Autodesk Inventor part; units mm, degrees
ref_plane "YZ Plane" through (0, 0, 0) normal (1, 0, 0) x (0, 1, 0)
ref_plane "XZ Plane" through (0, 0, 0) normal (0, 1, 0) x (-1, 0, 0)
ref_plane "XY Plane" through (0, 0, 0) normal (0, 0, 1) x (1, 0, 0)
ref_plane "Work Plane1" through (0, 0, 0) normal (0, 0, 1) x (1, 0, 0)
sketch "Sketch1" plane through (0, 0, 0) normal (0, 0, 1) x (1, 0, 0)
  circle A0 centre (44.9, 44.85) radius 3.1 construction
  arc A1 (2, 43.7546) -> (2, 45.9454) centre (4.9, 44.85) ccw construction
  line L0 (2, 39.7) -> (2, 43.7546) construction
  line L1 (97.8, 39.7) -> (2, 39.7) construction
  line L2 (97.8, 43.9046) -> (97.8, 39.7) construction
  arc A2 (94.119, 48) -> (97.8, 43.9046) centre (94.9, 45) ccw construction
  line L3 (55.681, 48) -> (94.119, 48) construction
  arc A3 (54.119, 48) -> (55.681, 48) centre (54.9, 45) ccw construction
  line L4 (29.1188, 48) -> (54.119, 48) construction
  line L5 (2, 45.9454) -> (2, 48) construction
  arc A4 (4.9, 2) -> (2, 5.7681) centre (4.9, 5) ccw construction
  line L6 (44.9, 2) -> (4.9, 2) construction
  circle A5 centre (44.9, 5) radius 3 construction
  line L7 (54.9, 2) -> (44.9, 2) construction
  circle A6 centre (54.9, 5) radius 3 construction
  line L8 (94.9, 2) -> (54.9, 2) construction
  arc A7 (97.8, 5.7681) -> (94.9, 2) centre (94.9, 5) ccw construction
  line L9 (97.8, 39.7) -> (97.8, 5.7681) construction
  line L10 (91.397, 39.7) -> (97.8, 39.7) construction
  line L11 (91.397, 10.3) -> (91.397, 39.7) construction
  line L12 (8.403, 10.3) -> (91.397, 10.3) construction
  line L13 (8.403, 10.3) -> (8.403, 39.7) construction
  line L14 (2, 39.7) -> (8.403, 39.7) construction
  line L15 (2, 5.7681) -> (2, 39.7) construction
  arc A8 (99.8, 48) -> (97.8, 50) centre (97.8, 48) ccw construction
  arc A9 (97.8, 0) -> (99.8, 2) centre (97.8, 2) ccw construction
  arc A10 (2, 50) -> (0, 48) centre (2, 48) ccw construction
  arc A11 (0, 2) -> (2, 0) centre (2, 2) ccw construction
  line L16 (0, 50) -> (99.8, 50)
  line L17 (99.8, 50) -> (99.8, 0)
  line L18 (99.8, 0) -> (0, 0)
  line L19 (0, 0) -> (0, 50)
  circle A12 centre (94.9, 45) radius 1.6 construction
  arc A13 (93.935, 3.8516) -> (95.865, 3.8516) centre (94.9, 5) ccw construction
  circle A14 centre (54.9, 5) radius 1.5 construction
  circle A15 centre (54.9, 45) radius 1.6 construction
  circle A16 centre (44.9, 44.85) radius 1.6 construction
  circle A17 centre (44.9, 5) radius 1.5 construction
  circle A18 centre (4.9, 44.85) radius 1.6 construction
  circle A19 centre (4.9, 5) radius 1.5 construction
  line L20 (0, 50) -> (50, 50) construction
  line L21 (50, 50) -> (50, 0) construction
  line L22 (50, 0) -> (0, 0) construction
  line L23 (0, 0) -> (0, 50) construction
  line L24 (50, 50) -> (0, 50)
  line L25 (0, 50) -> (0, 0)
  line L26 (0, 0) -> (50, 0)
  line L27 (50, 0) -> (50, 50)
  circle A20 centre (25, 25) radius 15
  circle A21 centre (44.9, 44.85) radius 1.5
  circle A22 centre (4.9, 44.85) radius 1.5
  circle A23 centre (4.9, 5) radius 1.5
  circle A24 centre (44.9, 5) radius 1.5
  line L28 (29.1188, 48) -> (29.1188, 47.25)
  line L29 (29.1188, 47.25) -> (20.2352, 47.25)
  line L30 (20.2352, 47.25) -> (20.2352, 48)
  line L31 (2, 48) -> (20.2352, 48)
  point P0 (0, 0)
  dimension "d0" = 50
  dimension "d1" = 50
  dimension "d2" = 30
  dimension "d3" = 3
  dimension "d4" = 3
  dimension "d5" = 3
  dimension "d6" = 3
extrude "Extrusion1" add sketch "Sketch1" along normal blind 2 contours L16 L27 L18 L19
sketch "Sketch2" plane through (0, 0, 2) normal (0, 0, 1) x (1, 0, 0)
  circle A0 centre (25, 25) radius 15
  circle A1 centre (44.9, 5) radius 1.5
  circle A2 centre (4.9, 5) radius 1.5
  circle A3 centre (4.9, 44.85) radius 1.5
  circle A4 centre (44.9, 44.85) radius 1.5
  line L0 (50, 50) -> (0, 50)
  line L1 (0, 50) -> (0, 0)
  line L2 (0, 0) -> (50, 0)
  line L3 (50, 0) -> (50, 50)
  circle A5 centre (25, 25) radius 15
  circle A6 centre (25, 25) radius 21
  point P0 (0, 0)
  dimension "d9" = 42
extrude "Extrusion2" add sketch "Sketch2" along normal blind 4.5 contours L3 L2 L1 L0
sketch "Sketch3" plane through (0, 0, 6.5) normal (0, 0, 1) x (1, 0, 0)
  point P0 (0, 0)
sketch "Sketch4" plane through (0, 0, 6.5) normal (0, 0, 1) x (1, 0, 0)
  arc A0 (5.5835, 17) -> (44.4165, 17) centre (25, 25) ccw construction
  line L0 (0.75, 17) -> (5.5835, 17) construction
  line L1 (0.75, 17) -> (0.75, 33) construction
  line L2 (5.5835, 33) -> (0.75, 33) construction
  arc A1 (44.4165, 33) -> (5.5835, 33) centre (25, 25) ccw construction
  line L3 (49.25, 33) -> (44.4165, 33) construction
  line L4 (49.25, 33) -> (49.25, 17) construction
  line L5 (44.4165, 17) -> (49.25, 17) construction
  line L6 (0, 0) -> (50, 0)
  line L7 (38.5, 50) -> (11.5, 50)
  line L8 (11.5, 50) -> (11.5, 0)
  line L9 (11.5, 0) -> (38.5, 0)
  line L10 (38.5, 0) -> (38.5, 50)
  line L11 (38.5, 50) -> (11.5, 0) construction
  line L12 (11.5, 50) -> (38.5, 0) construction
  line L13 (0, 50) -> (0, 0)
  line L14 (50, 38.5) -> (0, 38.5)
  line L15 (0, 38.5) -> (0, 11.5)
  line L16 (0, 11.5) -> (50, 11.5)
  line L17 (50, 11.5) -> (50, 38.5)
  line L18 (50, 38.5) -> (0, 11.5) construction
  line L19 (0, 38.5) -> (50, 11.5) construction
  circle A2 centre (4.9, 45) radius 0.6526
  circle A3 centre (44.9, 45) radius 0.6526
  circle A4 centre (4.9, 5) radius 0.6526
  circle A5 centre (44.9, 5) radius 0.6526
  line L20 (0, 0) -> (50, 0)
  line L21 (50, 0) -> (50, 50)
  line L22 (50, 50) -> (0, 50)
  line L23 (0, 50) -> (0, 0)
  dimension "d12" = 27
  dimension "d13" = 27
extrude "Extrusion3" cut sketch "Sketch4" against normal up to surface (4.5 mm away) contours L8 L16 L10 L6 | L13 L14 L8 L16 | L8 L14 L10 L16 | L10 L14 L17 L16 | L8 L7 L10 L14
properties part number "30_Z_Stage_Adapterplate"
Verification items for the finished model (mm, model axes). A direction names the side the tool comes from. Coordinates: 2 decimals unless noted, no trailing zeros. Order: outer loops, then holes, each group sorted by start corner. A loop starts at its lowest first (then second) coordinate and runs counter-clockwise, first axis right, second up. Notation, with made-up numbers: (19, 78) -> (48, 78) arc R24 cw to (48, 91) -> close; hole circle Ø2 at (-14.5, -30.5). An arc over 180 degrees is marked (long way). Put each result on its own line as item: value. Start each with the question number.
1. Access from +Z, -Z, +X, -X, +Y, -Y to the whole of each face (thin tool, end or side, straight path). Record for faces 4 (the flat face through (45, 11.5, 4)), 5 (the cylindrical face through (39.9, 10.2, 4.2)), 6 (the flat face through (36, 14, 0)), 7 (the flat face through (38.5, 4, 4)), 8 (the flat face through (6, 43, 6.5)).
2. Cross-section at B-B, the plane z = 4. Record the boundary of the cut face in (x, y), then the cut area to 3 significant figures.
3. Cross-section at C-C, the plane y = 13. Record the boundary of the cut face in (x, z).
4. Go/stop test with flat-tipped pins: pin 1 Ø1.5 at (x, y) = (43, 27) entering from +Z; pin 2 Ø2.5 at (x, y) = (4.9, 44.85) entering from -Z. Record where each tip stops, or that it passes through.
5. Cross-section at A-A, the plane x = 44.9. Record the boundary of the cut face in (y, z), then the cut area to 4 significant figures.
6. Cross-section at D-D, the plane x = 25. Record the boundary of the cut face in (y, z).
7. Material ranges on L1, parallel to Y at x = 4.9, z = 2.5; L2, parallel to Y at x = 44, z = 1.5; L3, parallel to Z at x = 34.5, y = 47.5, recorded low to high. Write a range as [from, to].
8. Mould release check, pull along Y, two halves, no side actions. Record for faces 1 (the cylindrical face through (10.2, 10.1, 4.2)), 2 (the flat face through (11.5, 5, 4)), 3 (the cylindrical face through (46.33, 4.55, 3.2)): released by +Y, released by -Y, zero draft, split by the parting line, or undercut.
Computed:
1. face 4: +Z, +X, -X
1. face 5: +Z
1. face 6: -Z, +X, -X, +Y, -Y
1. face 7: +Z, +Y, -Y
1. face 8: +Z, +X, -X, +Y, -Y
2. outline: (0, 0) -> (11.5, 0) -> (11.5, 8.91) arc R21 cw to (8.91, 11.5) -> (0, 11.5) -> close; (0, 38.5) -> (8.91, 38.5) arc R21 cw to (11.5, 41.09) -> (11.5, 50) -> (0, 50) -> close; (38.5, 0) -> (50, 0) -> (50, 11.5) -> (41.09, 11.5) arc R21 cw to (38.5, 8.91) -> close; (38.5, 41.09) arc R21 cw to (41.09, 38.5) -> (50, 38.5) -> (50, 50) -> (38.5, 50) -> close; hole circle Ø3 at (4.9, 5); hole circle Ø3 at (4.9, 44.85); hole circle Ø3 at (44.9, 5); hole circle Ø3 at (44.9, 44.85)
2. area: 487 mm2
3. outline: (0, 0) -> (16, 0) -> (16, 2) -> (0, 2) -> close; (34, 0) -> (50, 0) -> (50, 2) -> (34, 2) -> close
4. pin 1: z = 2
4. pin 2: through
5. outline: (0, 0) -> (3.5, 0) -> (3.5, 6.5) -> (0, 6.5) -> close; (6.5, 0) -> (43.35, 0) -> (43.35, 6.5) -> (38.5, 6.5) -> (38.5, 2) -> (11.5, 2) -> (11.5, 6.5) -> (6.5, 6.5) -> close; (46.35, 0) -> (50, 0) -> (50, 6.5) -> (46.35, 6.5) -> close
5. area: 164.5 mm2
6. outline: (0, 0) -> (10, 0) -> (10, 2) -> (0, 2) -> close; (40, 0) -> (50, 0) -> (50, 2) -> (40, 2) -> close
7. L1: [0, 3.5], [6.5, 11.5], [38.5, 43.35], [46.35, 50]
7. L2: [0, 3.8], [6.2, 43.65], [46.05, 50]
7. L3: [0, 2]
8. face 1: undercut
8. face 2: zero draft
8. face 3: undercut
